Work out the finished part from the listing and answer in its coordinate system (mm). Face numbers are marked on the shaded views. Round coordinates to 2 decimals unless told otherwise and drop trailing zeros. Order: outer loops, then holes, each group sorted by start corner. A loop starts at its lowest first (then second) coordinate and runs counter-clockwise, first axis right, second up. Notation, with made-up numbers: M 20,58 L 59,58 A10 ccw 59,71 Z; hole C 19,47 d11. An arc over 180 degrees is marked long. Return JSON: item names as keys, results as strings.
from build123d import *
from OCP.BRepFilletAPI import BRepFilletAPI_MakeChamfer

# Parameters (mm, degrees)
SKETCH2_R           = 4.7625
BOSS_EXTRUDE1_DEPTH = 11.1125
FILLET1_R           = 2.54
CHAMFER1_SIZE       = 5.08
CHAMFER1_SIZE2      = 1.84896879
FILLET2_R           = 1.27


with BuildPart() as part:
    # Sketch1 → Revolve1 (revolve)
    with BuildSketch(Plane(origin=(0, 0, 0), x_dir=(1, 0, 0), z_dir=(0, 1, 0)), mode=Mode.PRIVATE) as revolve1_sk:
        Polygon((-96.197401359, 18.174240066), (-96.197401359, 2.299240066), (2.227598641, 2.299240066), (2.227598641, 14.999240066), (78.427598641, 14.999240066), (78.427598641, 7.061740066), (81.602598641, 7.061740066), (81.602598641, 18.174240066), (-32.697401359, 18.174240066), (-32.697401359, 27.699240066), (-39.047401359, 27.699240066), (-39.047401359, 18.174240066), align=None)
    revolve(revolve1_sk.sketch.rotate(Axis((-96.197401359, 0, -2.299240066), (1, 0, 0)), 180), axis=Axis((-96.197401359, 0, -2.299240066), (1, 0, 0)))

    # Sketch2 → Boss-Extrude1 (add, symmetric)
    with BuildSketch(Plane(origin=(0, 0, 0), x_dir=(1, 0, 0), z_dir=(0, 1, 0))):
        with BuildLine():
            Line((-99.846730597, 9.692861011), (-96.197401359, 9.692861011))
            Line((-96.197401359, 9.692861011), (-96.197401359, -5.547138989))
            Line((-96.197401359, -5.547138989), (-100.132259318, -5.547138989))
            ThreePointArc((-100.132259318, -5.547138989), (-126.357394433, 2.566876274), (-99.846730597, 9.692861011))
        make_face()
        with Locations(Location((-112.072401359, 2.299240066, 0), (0, 0, 270))):
            Circle(SKETCH2_R, mode=Mode.SUBTRACT)
    extrude(amount=BOSS_EXTRUDE1_DEPTH, both=True)

    # Fillet1
    # the kernel refuses this fillet: 2.54 mm, written as the material it takes off along each edge
    with BuildSketch(Plane(origin=(-96.197401359, 0, -2.299240066), x_dir=(0, 0, 1), z_dir=(0, 1, 0))) as fillet1_piece_1_section:
        with BuildLine():
            CenterArc((15.875 - FILLET1_R, FILLET1_R), FILLET1_R, 270, 90)
            Line((15.875, FILLET1_R), (15.875, 0))
            Line((15.875, 0), (15.875 - FILLET1_R, 0))
        make_face()
    fillet1_piece_1 = revolve(axis=Axis((-96.197401359, 0, -2.299240066), (1, 0, 0)), mode=Mode.PRIVATE)
    fillet1_piece_1 = split(fillet1_piece_1, bisect_by=Plane(origin=(-95.476463438, -6.970916777, 5.547138989), z_dir=(0, 0, 1)), keep=Keep.TOP, mode=Mode.PRIVATE)
    add(fillet1_piece_1, mode=Mode.SUBTRACT)
    with BuildSketch(Plane(origin=(-96.197401359, 0, -2.299240066), x_dir=(0, 0, 1), z_dir=(0, 1, 0))) as fillet1_piece_2_section:
        with BuildLine():
            CenterArc((15.875 - FILLET1_R, FILLET1_R), FILLET1_R, 270, 90)
            Line((15.875, FILLET1_R), (15.875, 0))
            Line((15.875, 0), (15.875 - FILLET1_R, 0))
        make_face()
    fillet1_piece_2 = revolve(axis=Axis((-96.197401359, 0, -2.299240066), (1, 0, 0)), mode=Mode.PRIVATE)
    fillet1_piece_2 = split(fillet1_piece_2, bisect_by=Plane(origin=(-95.473294042, -11.1125, -2.089306166), z_dir=(0, -1, 0)), keep=Keep.TOP, mode=Mode.PRIVATE)
    add(fillet1_piece_2, mode=Mode.SUBTRACT)
    with BuildSketch(Plane(origin=(-96.197401359, 0, -2.299240066), x_dir=(0, 0, 1), z_dir=(0, 1, 0))) as fillet1_piece_3_section:
        with BuildLine():
            CenterArc((15.875 - FILLET1_R, FILLET1_R), FILLET1_R, 270, 90)
            Line((15.875, FILLET1_R), (15.875, 0))
            Line((15.875, 0), (15.875 - FILLET1_R, 0))
        make_face()
    fillet1_piece_3 = revolve(axis=Axis((-96.197401359, 0, -2.299240066), (1, 0, 0)), mode=Mode.PRIVATE)
    fillet1_piece_3 = split(fillet1_piece_3, bisect_by=Plane(origin=(-95.473294037, 11.1125, -2.089306166), z_dir=(0, 1, 0)), keep=Keep.TOP, mode=Mode.PRIVATE)
    add(fillet1_piece_3, mode=Mode.SUBTRACT)
    with BuildSketch(Plane(origin=(-96.197401359, 0, -2.299240066), x_dir=(0, 0, 1), z_dir=(0, 1, 0))) as fillet1_piece_4_section:
        with BuildLine():
            CenterArc((15.875 - FILLET1_R, FILLET1_R), FILLET1_R, 270, 90)
            Line((15.875, FILLET1_R), (15.875, 0))
            Line((15.875, 0), (15.875 - FILLET1_R, 0))
        make_face()
    fillet1_piece_4 = revolve(axis=Axis((-96.197401359, 0, -2.299240066), (1, 0, 0)), mode=Mode.PRIVATE)
    fillet1_piece_4 = split(fillet1_piece_4, bisect_by=Plane(origin=(-95.47646351, 0, -9.692861011), z_dir=(0, 0, -1)), keep=Keep.TOP, mode=Mode.PRIVATE)
    add(fillet1_piece_4, mode=Mode.SUBTRACT)

    # Chamfer1: one chamfer whose edges measure the first distance from different faces: ONE call of the kernel's chamfer builder (chamfer() names one face for all edges)
    chamfer1_edges_1 = [part.edges().sort_by_distance(p)[0] for p in [
        (-126.357394433, 11.1125, -2.566876274),
    ]]
    chamfer1_side_1 = [part.faces().sort_by_distance(p)[0] for p in [
        (-125.941875569, 11.1125, -2.559091328),
    ]]
    chamfer1_edges_2 = [part.edges().sort_by_distance(p)[0] for p in [
        (-126.357394433, -11.1125, -2.566876274),
    ]]
    chamfer1_side_2 = [part.faces().sort_by_distance(p)[0] for p in [
        (-125.941875569, -11.1125, -2.559091328),
    ]]
    chamfer1 = BRepFilletAPI_MakeChamfer(part.part.solid().wrapped)
    for e in chamfer1_edges_1:
        chamfer1.Add(CHAMFER1_SIZE, CHAMFER1_SIZE2, e.wrapped, chamfer1_side_1[0].wrapped)  # the first distance lies on this face
    for e in chamfer1_edges_2:
        chamfer1.Add(CHAMFER1_SIZE, CHAMFER1_SIZE2, e.wrapped, chamfer1_side_2[0].wrapped)  # the first distance lies on this face
    add(Compound.cast(chamfer1.Shape()), mode=Mode.REPLACE)

    # Fillet2
    fillet2_edges = [part.edges().sort_by_distance(p)[0] for p in [
        (81.602598641, 0, -18.174240066),
    ]]
    fillet(fillet2_edges, radius=FILLET2_R)


solid = part.part
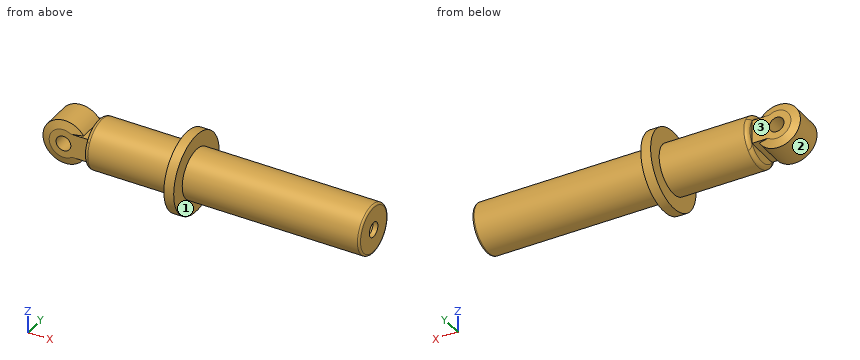
Item 1: Find section D-D (z = -20.5). Determine the outline of the cut face in (x, y).
Output:
{"outline": "M -39.05,-17.72 L -32.7,-17.72 L -32.7,17.72 L -39.05,17.72 Z"}
Item 2: Find section A-A (x = 29.5). Determine the outline of the cut face in (y, z) (3 decimals), plus the area to 3 significant figures.
Output:
{"outline": "C 0,-2.299 d31.75; hole C 0,-2.299 d25.4", "area": "285 mm^2"}
Item 3: Each of these flat-tipped pins is pushed along its axis until it touches: pin 1 (9 mm diameter, centred on x = -100, y = -3.5, fed in from +Z); pin 2 (5 mm diameter, centred on x = -88.5, z = -8.5, fed in from +Y); pin 3 (1.5 mm diameter, centred on y = 5.5, z = 9, fed in from -X); pin 4 (15 mm diameter, centred on y = -1, z = -1.5, fed in from +X). Where does it stop, or does it pass through?
Output:
{"pin 1": "stops at z = 12.46", "pin 2": "stops at y = 15.44", "pin 3": "stops at x = -121.71", "pin 4": "stops at x = 81.6"}
Item 4: The mould has two halves that part along X. Classify the marked faces 1, 2 and 3: pulls with the +X half, pulls with the -X half, needs draft (parallel to the pull), parting line crosses it, or undercut.
Output:
{"face 1": "pulls with the +X half", "face 2": "undercut", "face 3": "needs draft"}
Item 5: Find section C-C (x = -3.5). Determine the outline of the cut face in (y, z) (3 decimals), plus the area to 3 significant figures.
Output:
{"outline": "C 0,-2.299 d31.75", "area": "792 mm^2"}
Item 6: Consider line 1 along X through (y, z) = (-5.5, 2); line 2 along X through (y, z) = (4, -18.5); line 3 along Y through (x, z) = (-40, -2). Determine where each line is inside the solid, lowest interval first. Write a range as [from, to].
Output:
{"line 1": "x = [-125.7, -114.12], [-110.02, 2.23], [78.43, 81.6]", "line 2": "x = [-39.05, -32.7]", "line 3": "y = [-15.87, 15.87]"}
